```python
from build123d import *

# Parameters (mm, degrees)
SKETCH_7_R          = 17
EXTRUDE_6_DEPTH     = 15
SKETCH_8_R          = 1.5
CUT_EXTRUDE_2_DEPTH = 5
SKETCH_9_R          = 2
EXTRUDE_7_DEPTH     = 3.5


with BuildPart() as part:
    # Эскиз7 → Бобышка-Вытянуть6 (new body)
    with BuildSketch(Plane(origin=(0, 0, 0), x_dir=(1, 0, 0), z_dir=(0, 1, 0))):
        with Locations(Location((0, 0, 0), (0, 0, 270))):
            Circle(SKETCH_7_R)
    extrude(amount=EXTRUDE_6_DEPTH)

    # Эскиз8 → Вырез-Вытянуть2 (cut)
    with BuildSketch(Plane.XZ):
        with Locations(Location((-5.1, 8.833459119, 0), (0, 0, 270))):
            Circle(SKETCH_8_R)
        with Locations(Location((5.1, 8.833459119, 0), (0, 0, 270))):
            Circle(SKETCH_8_R)
        with Locations(Location((-10.2, 0, 0), (0, 0, 270))):
            Circle(SKETCH_8_R)
        with Locations(Location((-5.1, -8.833459119, 0), (0, 0, 270))):
            Circle(SKETCH_8_R)
        with Locations(Location((10.2, 0, 0), (0, 0, 270))):
            Circle(SKETCH_8_R)
        with Locations(Location((5.1, -8.833459119, 0), (0, 0, 270))):
            Circle(SKETCH_8_R)
    extrude(amount=-CUT_EXTRUDE_2_DEPTH, mode=Mode.SUBTRACT)

    # Эскиз9 → Бобышка-Вытянуть7 (add)
    with BuildSketch(Plane.XZ):
        with Locations(Location((8.660254038, 5, 0), (0, 0, 270))):
            Circle(SKETCH_9_R)
        with Locations(Location((0, -10, 0), (0, 0, 90))):
            Circle(SKETCH_9_R)
        with Locations(Location((-8.660254038, 5, 0), (0, 0, 90))):
            Circle(SKETCH_9_R)
    extrude(amount=EXTRUDE_7_DEPTH)


solid = part.part
```
Build history of the part. All positions in model axes, mm. A direction names the side the tool comes from. Coordinates: 2 decimals unless noted, no trailing zeros. Write each loop counter-clockwise with the first axis right and the second up, starting at its lowest first coordinate (ties: lowest second). Pieces come first, ordered by that corner, then holes.
1. Pull direction Z, two halves, no side cores. Call faces 1 (the cylindrical face through (-11.664, 2.465, 0.325)), 2 (the flat face through (-10, 5, 0)), 3 (the flat face through (9, -3.5, 5)), 4 (the cylindrical face through (16.855, 7.395, -2.213)): released by +Z, released by -Z, zero draft, split by the parting line, or undercut.
Answer block:
face 1: undercut
face 2: undercut
face 3: zero draft
face 4: split by the parting line
2. Drop flat-ended pins along their axis: pin 1 (0.9 mm diameter, centred on x = -5, z = -9, fed in from -Y); pin 2 (5 mm diameter, centred on x = -5.1, z = 8.83, fed in from -Y); pin 3 (8 mm diameter, centred on x = 10, y = 2.5, fed in from -Z). Give the stop position or say it passes through.
Answer block:
pin 1: stops at y = 5
pin 2: stops at y = 0
pin 3: stops at z = -15.91
3. Band-saw the part on D-D, the plane z = 5. Give the cut face in (x, y), and give its area (3 significant figures).
Answer block:
outline: (-16.25, 0) - (-10.66, 0) - (-10.66, -3.5) - (-6.66, -3.5) - (-6.66, 0) - (6.66, 0) - (6.66, -3.5) - (10.66, -3.5) - (10.66, 0) - (16.25, 0) - (16.25, 15) - (-16.25, 15) - close
area: 515 mm2
4. Drill centre lines: probe 1 along X at (y, z) = (3.25, 0); probe 2 along X at (y, z) = (1.5, -9); probe 3 along Y at (x, z) = (12.5, 8). Where is each one in solid material? Low to high.
Answer block:
probe 1: x = -17 to -11.7, -8.7 to 8.7, 11.7 to 17
probe 2: x = -14.42 to -6.59, -3.61 to 3.61, 6.59 to 14.42
probe 3: y = 0 to 15
5. Band-saw the part on A-A, the plane z = 0. Give the cut face in (x, y), and give its area (3 significant figures).
Answer block:
outline: (-17, 0) - (-11.7, 0) - (-11.7, 5) - (-8.7, 5) - (-8.7, 0) - (8.7, 0) - (8.7, 5) - (11.7, 5) - (11.7, 0) - (17, 0) - (17, 15) - (-17, 15) - close
area: 480 mm2
6. Band-saw the part on B-B, the plane x = 0. Give the cut face in (y, z).
Answer block:
outline: (-3.5, -12) - (0, -12) - (0, -17) - (15, -17) - (15, 17) - (0, 17) - (0, -8) - (-3.5, -8) - close
7. 3-axis set-ups, long thin cutter, end or side, ignore diameter. For faces 5 (the flat face through (-9, -3.5, 5)), 6 (the cylindrical face through (4.53, 2.46, -10.22)): which of +Z, -Z, +X, -X, +Y, -Y reach the whole face in a straight line?
Answer block:
face 5: +Z, -Z, +X, -X, -Y
face 6: -Y
8. Band-saw the part on C-C, the plane y = 7.75. Give the cut face in (x, z), and give its area (3 significant figures).
Answer block:
outline: circle Ø34 at (0, 0)
area: 908 mm2
